from build123d import *

# Parameters (mm, degrees)
BOSS_EXTRUDE1_DEPTH = 30
SKETCH2_W           = 30
SKETCH2_H           = 45
BOSS_EXTRUDE2_DEPTH = 10
SKETCH3_W           = 15
SKETCH3_H           = 10
BOSS_EXTRUDE3_DEPTH = 5
CUT_EXTRUDE1_DEPTH  = 15
CUT_EXTRUDE2_DEPTH  = 12
SKETCH6_W           = 5
SKETCH6_H           = 10
CUT_EXTRUDE4_DEPTH  = 67.098411479


with BuildPart() as part:
    # Sketch1 → Boss-Extrude1 (new body)
    with BuildSketch(Plane(origin=(0, 0, 0), x_dir=(1, 0, 0), z_dir=(0, 1, 0))):
        Polygon((0, 0), (38, 0), (38, -5), (30, -5), (5, -20), (0, -20), align=None)
    extrude(amount=BOSS_EXTRUDE1_DEPTH)

    # Sketch2 → Boss-Extrude2 (add)
    with BuildSketch(Plane(origin=(0, 0, 0), x_dir=(1, 0, 0), z_dir=(0, 1, 0))):
        with Locations((15, -22.5)):
            Rectangle(SKETCH2_W, SKETCH2_H)
    extrude(amount=BOSS_EXTRUDE2_DEPTH)

    # Sketch3 → Boss-Extrude3 (add)
    with BuildSketch(Plane(origin=(0, 0, 0), x_dir=(0, 0, -1), z_dir=(1, 0, 0))):
        with Locations((-27.5, 15)):
            Rectangle(SKETCH3_W, SKETCH3_H)
    extrude(amount=BOSS_EXTRUDE3_DEPTH)

    # Sketch4 → Cut-Extrude1 (cut)
    with BuildSketch(Plane(origin=(0, 30, 0), x_dir=(1, 0, 0), z_dir=(0, 1, 0))):
        Polygon((30, -5), (15, -5), (15, -14), align=None)
    extrude(amount=-CUT_EXTRUDE1_DEPTH, mode=Mode.SUBTRACT)

    # Sketch5 → Cut-Extrude2 (cut)
    with BuildSketch(Plane(origin=(30, 0, 0), x_dir=(0, 0, -1), z_dir=(1, 0, 0))):
        Polygon((-45, 10), (-45, 0), (-29, 10), align=None)
    extrude(amount=-CUT_EXTRUDE2_DEPTH, mode=Mode.SUBTRACT)

    # Sketch6 → Cut-Extrude4 (cut, through all)
    with BuildSketch(Plane(origin=(0, 0, 0), x_dir=(1, 0, 0), z_dir=(0, 1, 0))):
        with Locations((27.5, -40)):
            Rectangle(SKETCH6_W, SKETCH6_H)
    extrude(amount=CUT_EXTRUDE4_DEPTH, mode=Mode.SUBTRACT)


solid = part.part
The model under review builds one solid part; all positions refer to its coordinate system, in mm. A direction names the side the tool comes from. Give positions to 0.01 mm unless a question says otherwise; leave off trailing zeros. Loops run counter-clockwise (first coordinate to the right, second up) from the corner with the lowest first, then second, coordinate; pieces in that order, holes last. Notation, with made-up numbers: (21, 15) -> (32, 15) arc R21 ccw to (32, 35) -> close; hole circle Ø2 at (25, 12). An arc over 180 degrees is marked (long way). Put each result on its own line as item: value. Start each with the question number.
1. We need section C-C on z = 27.5. State the section outline as (x, y) points, then the cut area to 3 significant figures.
2. We need section B-B on x = 23. State the section outline as (y, z) points, then the cut area to 3 significant figures.
3. For faces 1 (the face through (0, 12, 18)), 2 (the face through (27, 3, 35)), 3 (the face through (2, 15, 35)), 4 (the face through (11, 30, 8)), 5 (the face through (21, 15, 8)), list the 3-axis set-ups (+Z, -Z, +X, -X, +Y, -Y) from which the entire face can be reached by the end or side of a thin tool; tool diameter is ignored.
4. Wall thickness on probe 1 along X at (y, z) = (10.25, 21.5); probe 2 along X at (y, z) = (9.5, 32); probe 3 along Y at (x, z) = (19.5, 24): over which ranges is each line inside the solid? List them lowest first.
5. We need section A-A on y = 13.5. State the section outline as (x, z) points, then the cut area to 4 significant figures.
6. Clearance check with flat-ended pins moving along their axes: P1, Ø8, axis at x = 28, z = 14, coming from the +Y side; P2, Ø5, axis at y = 2.5, z = 42, coming from the +X side; P3, Ø1.5, axis at y = 23, z = 8.5, coming from the +X side. State where each tip first meets the part, or that it passes through.
7. We need section D-D on x = 2.5. State the section outline as (y, z) points, then the cut area to 3 significant figures.
Determined:
1. outline: (0, 0) -> (30, 0) -> (30, 10) -> (5, 10) -> (5, 20) -> (0, 20) -> close
1. area: 350 mm^2
2. outline: (0, 0) -> (30, 0) -> (30, 5) -> (15, 5) -> (15, 9.2) -> (10, 9.2) -> (10, 29) -> (0, 45) -> close
2. area: 491 mm^2
3. face 1: +Z, -Z, -X, +Y, -Y
3. face 2: +Z, +X, +Y, -Y
3. face 3: +Z, +X, -X, +Y
3. face 4: +Z, -Z, +X, -X, +Y
3. face 5: +Z, +X, +Y
4. probe 1: 0 to 5
4. probe 2: 0 to 18
4. probe 3: 0 to 10
5. outline: (0, 0) -> (38, 0) -> (38, 5) -> (30, 5) -> (5, 20) -> (5, 35) -> (0, 35) -> close
5. area: 527.5 mm^2
6. P1: y = 10
6. P2: x = 25
6. P3: x = 15
7. outline: (0, 0) -> (30, 0) -> (30, 20) -> (20, 20) -> (20, 35) -> (10, 35) -> (10, 45) -> (0, 45) -> close
7. area: 1,000 mm^2
